```python
from build123d import *

# Parameters (mm, degrees)
BOSS_EXTRUDE1_DEPTH                                  = 250
CSK_FOR_M4_HEX_SOCKET_COUNTERSUNK_HEAD_S_D           = 4.5
CSK_FOR_M4_HEX_SOCKET_COUNTERSUNK_HEAD_S_DEPTH       = 5.4
CSK_FOR_M4_HEX_SOCKET_COUNTERSUNK_HEAD_S_CSINK_D     = 9.18
CSK_FOR_M4_HEX_SOCKET_COUNTERSUNK_HEAD_S_CSINK_ANGLE = 90
CSK_FOR_M4_HEX_SOCKET_COUNTERSUNK_HEAD_S_TIP         = 1.351936393


with BuildPart() as part:
    # Sketch1 → Boss-Extrude1 (new, symmetric)
    with BuildSketch(Plane(origin=(0, 0, 0), x_dir=(0, 0, -1), z_dir=(1, 0, 0))):
        Polygon((-4.75, 4.75), (-9.5, 4.75), (-9.5, -4.75), (9.5, -4.75), (9.5, 4.75), (4.75, 4.75), (4.75, 1.9), (7.1, 1.9), (7.1, -1.4), (4.75, -1.4), (4.75, -1.9), (-4.75, -1.9), (-4.75, -1.4), (-7.1, -1.4), (-7.1, 1.9), (-4.75, 1.9), align=None)
    extrude(amount=BOSS_EXTRUDE1_DEPTH, both=True)

    # CSK for M4 Hex Socket Countersunk Head Screw1
    with Locations(Plane(origin=(0, -1.9, 0), x_dir=(1, 0, 0), z_dir=(0, 1, 0))):
        with Locations((0, 0), (-210, 0), (210, 0)):
            CounterSinkHole(CSK_FOR_M4_HEX_SOCKET_COUNTERSUNK_HEAD_S_D / 2, CSK_FOR_M4_HEX_SOCKET_COUNTERSUNK_HEAD_S_CSINK_D / 2, depth=CSK_FOR_M4_HEX_SOCKET_COUNTERSUNK_HEAD_S_DEPTH, counter_sink_angle=CSK_FOR_M4_HEX_SOCKET_COUNTERSUNK_HEAD_S_CSINK_ANGLE)
            with Locations((0, 0, -(CSK_FOR_M4_HEX_SOCKET_COUNTERSUNK_HEAD_S_DEPTH + CSK_FOR_M4_HEX_SOCKET_COUNTERSUNK_HEAD_S_TIP / 2))):  # 118° drill point
                Cone(0, CSK_FOR_M4_HEX_SOCKET_COUNTERSUNK_HEAD_S_D / 2, CSK_FOR_M4_HEX_SOCKET_COUNTERSUNK_HEAD_S_TIP, mode=Mode.SUBTRACT)


solid = part.part
```
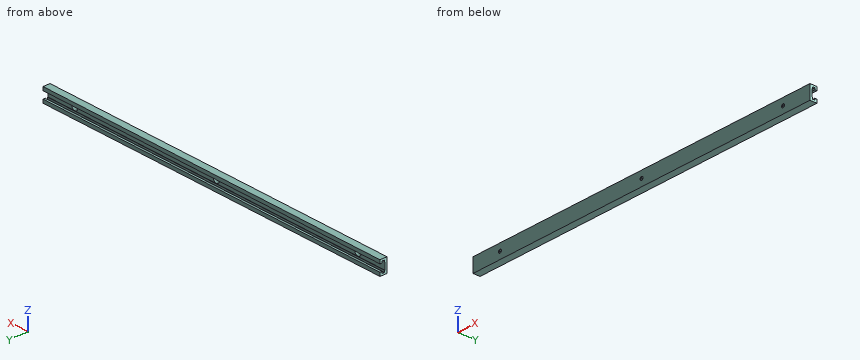
Model file for the job. Use its own axes, mm. Give positions to 0.01 mm unless a question says otherwise; leave off trailing zeros. Write each loop counter-clockwise with the first axis right and the second up, starting at its lowest first coordinate (ties: lowest second). Pieces come first, ordered by that corner, then holes. Notation, with made-up numbers: (59.5, -31.75) -> (68.5, -31.75) arc R20 cw to (68.5, -17.75) -> close; hole circle Ø5 at (-31.75, 38). An arc over 180 degrees is marked (long way). Use CSV: the item, a comma, the result in double quotes. Start each with the question number.
1) Drill centre lines: L1, parallel to Z at x = 48.5, y = 2.25; L2, parallel to Z at x = -210, y = -4.5; L3, parallel to Y at x = -68.5, z = -3.25. Where is each one in solid material? Low to high.
2) Cut at B-B on x = -149.5. List the corners of the cut face in (y, z), plus the area to 3 significant figures.
3) Cut at A-A on y = 0.25. List the corners of the cut face in (x, z), plus the area to 3 significant figures.
Final values:
1,L1,"z = -9.5 to -4.75, 4.75 to 9.5"
1,L2,"z = -9.5 to -2.25, 2.25 to 9.5"
1,L3,"y = -4.75 to -1.9"
2,outline,"(-4.75, -9.5) -> (4.75, -9.5) -> (4.75, -4.75) -> (1.9, -4.75) -> (1.9, -7.1) -> (-1.4, -7.1) -> (-1.4, -4.75) -> (-1.9, -4.75) -> (-1.9, 4.75) -> (-1.4, 4.75) -> (-1.4, 7.1) -> (1.9, 7.1) -> (1.9, 4.75) -> (4.75, 4.75) -> (4.75, 9.5) -> (-4.75, 9.5) -> close"
2,area,"102 mm2"
3,outline,"(-250, -9.5) -> (250, -9.5) -> (250, -7.1) -> (-250, -7.1) -> close; (-250, 7.1) -> (250, 7.1) -> (250, 9.5) -> (-250, 9.5) -> close"
3,area,"2,400 mm2"
